Part model, mm, in its own coordinate system. Face numbers are marked on the shaded views. Round coordinates to 2 decimals unless told otherwise and drop trailing zeros. Write each loop counter-clockwise with the first axis right and the second up, starting at its lowest first coordinate (ties: lowest second). Pieces come first, ordered by that corner, then holes.
```python
from build123d import *

# Parameters (mm, degrees)
ESQUISSE1_R                     = 25
ESQUISSE1_R_2                   = 24
BOSS_EXTRU_1_DEPTH              = 30
ESQUISSE2_R                     = 32
ESQUISSE2_R_2                   = 25
BOSS_EXTRU_2_DEPTH              = 30
ESQUISSE3_R                     = 35
ESQUISSE3_R_2                   = 25
ENL_V_DE_MAT_EXTRU_MINCE1_DEPTH = 0.5
CONG_1_R                        = 4


with BuildPart() as part:
    # Esquisse1 → Boss.-Extru.1 (new body)
    with BuildSketch(Plane.XY):
        Circle(ESQUISSE1_R)
        Circle(ESQUISSE1_R_2, mode=Mode.SUBTRACT)
    extrude(amount=BOSS_EXTRU_1_DEPTH)

    # Esquisse2 → Boss.-Extru.2 (add)
    with BuildSketch(Plane.XY.offset(30)):
        Circle(ESQUISSE2_R)
        Circle(ESQUISSE2_R_2, mode=Mode.SUBTRACT)
    extrude(amount=-BOSS_EXTRU_2_DEPTH)

    # Esquisse3 → Enlèv. de mat.-Extru.-Mince1 (cut)
    with BuildSketch(Plane.XY.offset(30)):
        Circle(ESQUISSE3_R)
        Circle(ESQUISSE3_R_2, mode=Mode.SUBTRACT)
    enl_v_de_mat_extru_mince1 = extrude(amount=-ENL_V_DE_MAT_EXTRU_MINCE1_DEPTH, mode=Mode.SUBTRACT)

    # Symétrie1: Enlèv. de mat.-Extru.-Mince1 across plane
    add(enl_v_de_mat_extru_mince1.mirror(Plane.XY.offset(15)), mode=Mode.SUBTRACT)

    # Congé1
    cong_1_edges = [part.edges().sort_by_distance(p)[0] for p in [
        (-32, 0, 29.5),
        (-32, 0, 0.5),
    ]]
    fillet(cong_1_edges, radius=CONG_1_R)


solid = part.part
```
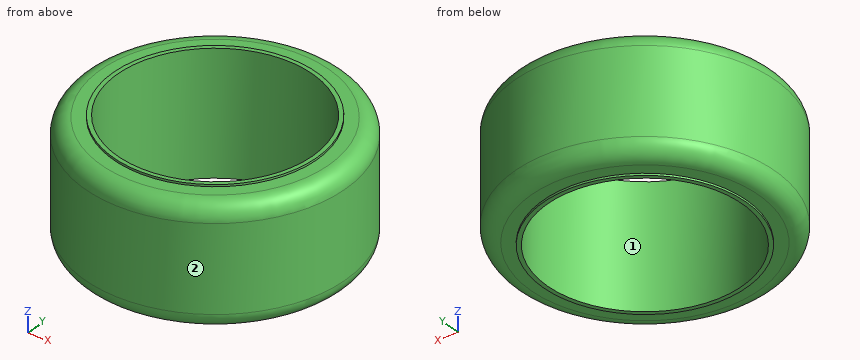
Q1. Cut at C-C on z = 18. Write the cut outline in (x, y), plus the area to 3 significant figures.
Values follow:
outline: circle Ø64 at (0, 0); hole circle Ø48 at (0, 0)
area: 1,410 mm2
Q2. Wall check: L1, parallel to Y at x = 0, z = 14; L2, parallel to Y at x = 5.5, z = 17.25; L3, parallel to X at y = -7, z = 21.25. Give the ranges that are in metal, low to high.
Values follow:
L1: y = -32 to -24, 24 to 32
L2: y = -31.52 to -23.36, 23.36 to 31.52
L3: x = -31.22 to -22.96, 22.96 to 31.22
Q3. Drop flat-ended pins along their axis: pin 1 (12 mm diameter, centred on x = -11.5, z = 12, fed in from -Y); pin 2 (5 mm diameter, centred on y = -18, z = 10, fed in from -X); pin 3 (5 mm diameter, centred on x = -3, z = 15, fed in from +Y). Give the stop position or say it passes through.
Values follow:
pin 1: stops at y = -31.52
pin 2: stops at x = -28
pin 3: stops at y = 32
Q4. Cut at A-A on x = 0. Write the cut outline in (y, z).
Values follow:
outline: (-32, 4.5) arc R4 ccw to (-28, 0.5) - (-25, 0.5) - (-25, 0) - (-24, 0) - (-24, 30) - (-25, 30) - (-25, 29.5) - (-28, 29.5) arc R4 ccw to (-32, 25.5) - close; (24, 0) - (25, 0) - (25, 0.5) - (28, 0.5) arc R4 ccw to (32, 4.5) - (32, 25.5) arc R4 ccw to (28, 29.5) - (25, 29.5) - (25, 30) - (24, 30) - close
Q5. Mould opens along Y. For the marked faces 1 and 2 say: +Y half, -Y half, draft (parallel to the pull), parting line (faces both ways), or undercut.
Values follow:
face 1: undercut
face 2: parting line
